Design review of the part built by this model. Coordinates are the model's own, in mm. Face numbers are marked on the shaded views. A direction names the side the tool comes from. Give positions to 0.01 mm unless a question says otherwise; leave off trailing zeros. Write each loop counter-clockwise with the first axis right and the second up, starting at its lowest first coordinate (ties: lowest second). Pieces come first, ordered by that corner, then holes.
```python
from build123d import *

# Parameters (mm, degrees)
F0_W      = 203.2
F0_H      = 454.152
F1_DEPTH  = 25.4
F2_W      = 6.35
F2_H      = 152.4
F3_DEPTH  = 203.201
F4_W      = 457.2
F4_H      = 203.2
F5_DEPTH  = 12.7
F6_W      = 127
F6_H      = 190.5
F7_DEPTH  = 9.652
F9_D      = 11.1125
F11_DEPTH = 4.7625
F12_W     = 38.1
F12_H     = 38.1
F13_DEPTH = 203.201
F15_D     = 17.4625
F17_DEPTH = 4.826


# Not quite as in the source:
# - a length typed as a fraction of an inch, garbled in the dataset ("3 / 203.2 mm" for 3/8 in), is restored


with BuildPart() as f1:
    # F0 (on Right) → F1 (new body)
    with BuildSketch(Plane.YZ):
        Rectangle(F0_W, F0_H)
    extrude(amount=F1_DEPTH)

    # F2 (on face) → F3 (cut, through all)
    with BuildSketch(Plane.XZ.offset(101.6)):
        with Locations((3.175, -150.876)):
            Rectangle(F2_W, F2_H)
    extrude(amount=-F3_DEPTH, mode=Mode.SUBTRACT)

    # F4 (on face) → F5 (join)
    with BuildSketch(Plane.XY.offset(227.076)):
        with Locations((95.25, 0)):
            Rectangle(F4_W, F4_H)
    extrude(amount=F5_DEPTH)

    # F6 (on face) → F7 (join)
    with BuildSketch(Plane.XY.offset(239.776)):
        with Locations((-63.5, 0)):
            Rectangle(F6_W, F6_H)
        with Locations((254, 0)):
            Rectangle(F6_W, F6_H)
    extrude(amount=F7_DEPTH)

    # F9 (through all)
    with Locations(Plane.XY.offset(249.428)):
        with Locations((-101.6, 61.976), (-25.4, 61.976), (-101.6, -61.976), (-25.4, -61.976), (215.9, 61.976), (292.1, 61.976), (215.9, -61.976), (292.1, -61.976)):
            Hole(F9_D / 2)

    # F10 (on Front) → F11 (join, symmetric)
    with BuildSketch(Plane.XZ):
        Polygon((317.5, 227.076), (25.4, 227.076), (25.4, -227.076), (50.8, -227.076), (317.5, 201.676), align=None)
    extrude(amount=F11_DEPTH, both=True)

    # F12 (on face) → F13 (cut, through all)
    with BuildSketch(Plane.XZ.offset(101.6)):
        with Locations((-5.842, -169.672)):
            Rectangle(F12_W, F12_H)
    extrude(amount=-F13_DEPTH, mode=Mode.SUBTRACT)

    # F15 (through all)
    with Locations(Plane(origin=(6.35, 0, 0), x_dir=(0, -1, 0), z_dir=(-1, 0, 0))):
        with Locations((-82.55, -131.572), (82.55, -131.572), (82.55, -207.772), (-82.55, -207.772)):
            Hole(F15_D / 2)

    # F16 (on Front) → F17 (join, symmetric)
    with BuildSketch(Plane.XZ):
        Polygon((0, 100.076), (0, 227.076), (-127, 227.076), (-127, 201.676), (-25.4, 100.076), align=None)
    extrude(amount=F17_DEPTH, both=True)


solid = f1.part
```
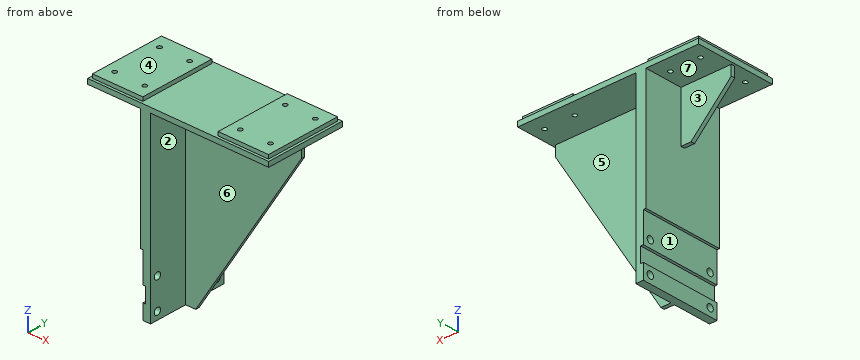
(1) To check wall thickness, follow L1, parallel to Z at x = 13.75, y = 82.55; L2, parallel to Y at x = -101, z = 236; L3, parallel to Y at x = -101.6, z = 232.25. State the ranges of each line that lie inside material, in increasing order.
Resolved:
L1: z = -227.08 to -216.5, -199.04 to -140.3, -122.84 to 239.78
L2: y = -101.6 to -67.5, -56.45 to 56.45, 67.5 to 101.6
L3: y = -101.6 to -67.53, -56.42 to 56.42, 67.53 to 101.6
(2) Consider section D-D, the plane z = -108. Give the boundary of the cut face in (x, y).
Resolved:
outline: (6.35, -101.6) - (25.4, -101.6) - (25.4, -4.76) - (124.87, -4.76) - (124.87, 4.76) - (25.4, 4.76) - (25.4, 101.6) - (6.35, 101.6) - close
(3) Consider section A-A, the plane y = 82.55. Give the number of separate pieces and of enclosed holes in the cut face, then the cut area to 3 significant figures.
Resolved:
separate pieces: 3
enclosed holes: 0
area: 17,900 mm2
(4) Consider section C-C, the plane y = -23. Give the boundary of the cut face in (x, z).
Resolved:
outline: (-133.35, 227.08) - (0, 227.08) - (0, -74.68) - (6.35, -74.68) - (6.35, -150.62) - (13.21, -150.62) - (13.21, -188.72) - (6.35, -188.72) - (6.35, -227.08) - (25.4, -227.08) - (25.4, 227.08) - (323.85, 227.08) - (323.85, 239.78) - (317.5, 239.78) - (317.5, 249.43) - (190.5, 249.43) - (190.5, 239.78) - (0, 239.78) - (0, 249.43) - (-127, 249.43) - (-127, 239.78) - (-133.35, 239.78) - close
(5) Consider section B-B, the plane x = 292.1. Give the boundary of the cut face in (y, z), then the cut area to 3 significant figures.
Resolved:
outline: (-101.6, 227.08) - (-67.53, 227.08) - (-67.53, 249.43) - (-95.25, 249.43) - (-95.25, 239.78) - (-101.6, 239.78) - close; (-56.42, 227.08) - (-4.76, 227.08) - (-4.76, 160.84) - (4.76, 160.84) - (4.76, 227.08) - (56.42, 227.08) - (56.42, 249.43) - (-56.42, 249.43) - close; (67.53, 227.08) - (101.6, 227.08) - (101.6, 239.78) - (95.25, 239.78) - (95.25, 249.43) - (67.53, 249.43) - close
area: 4,550 mm2
(6) Tool access review of the marked faces 1, 2, 3 and 4: name each direction out of +Z, -Z, +X, -X, +Y, -Y from which nothing blocks a thin tool from reaching the whole face with its end or side.
Resolved:
face 1: -Z, -X, +Y, -Y
face 2: -Z, +X, -Y
face 3: -Z, -X, +Y
face 4: +Z, +X, -X, +Y, -Y
(7) Mouldability with a two-part tool opening along Y and no side actions: class the marked faces 5, 6 and 7 as pulls with the +Y half, pulls with the -Y half, needs draft (parallel to the pull), parting line crosses it, or undercut.
Resolved:
face 5: pulls with the +Y half
face 6: pulls with the -Y half
face 7: needs draft
(8) Clearance check with flat-ended pins moving along their axes: P1, Ø5, axis at y = 4, z = -31, coming from the +X side; P2, Ø3, axis at x = 240, z = 246.5, coming from the +Y side; P3, Ø5, axis at y = 22, z = 246, coming from the +X side. State where each tip first meets the part, or that it passes through.
Resolved:
P1: stops at x = 174.32
P2: stops at y = 95.25
P3: stops at x = 317.5
